Read the model definition and answer for the solid it produces. Units are mm, in the model's axes. Coordinates: 2 decimals unless noted, no trailing zeros. Order: outer loops, then holes, each group sorted by start corner. A loop starts at its lowest first (then second) coordinate and runs counter-clockwise, first axis right, second up. Notation, with made-up numbers: M 42,-6 L 79,-6 A34 ccw 79,31 Z; hole C 33.25,-26.75 d9. An arc over 180 degrees is marked long. One line per question, with ' | ' between items. Start each with the question number.
1) Consider probe 1 along Y at (x, z) = (0, 1.65); probe 2 along X at (y, z) = (-2.5, 1.5); probe 3 along X at (y, z) = (-3, 2.3). Determine where each line is inside the solid, lowest interval first.
2) Find section B-B, the plane x = 27. Write down the section's boundary in (y, z).
3) Find section A-A, the plane y = 33.5. Write down the section's boundary in (x, z), plus the area to 3 significant figures.
4) Find section C-C, the plane z = 1.45. Write down the section's boundary in (x, y).
5) Find section D-D, the plane y = -14.5. Write down the section's boundary in (x, z), plus the area to 3 significant figures.
6) Given P1, Ø16, axis at x = 27, y = 0, coming from the -Z side; P2, Ø1.5, axis at x = -8.5, z = 2, coming from the +Y side; P3, Ø1.5, axis at x = -7, z = 2, coming from the +Y side; P4, Ø1.5, axis at y = 10, z = 0.5, coming from the +X side, each flat-ended and moving along its own axis, determine where each tip first touches the part or whether it passes through.
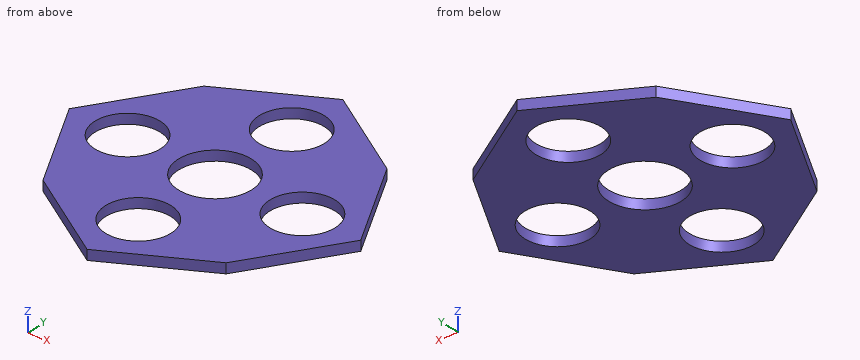
from build123d import *

# Parameters (mm, degrees)
F0_R     = 9.85
F0_R_2   = 11
F1_DEPTH = 3


with BuildPart() as f1:
    # F0 (on Top) → F1 (new body)
    with BuildSketch(Plane.XY):
        Polygon((-28.284271, 28.284271), (-45, 0), (-28.284271, -28.284271), (0, -45), (28.284271, -28.284271), (45, 0), (28.284271, 28.284271), (0, 45), align=None)
        with Locations((0, -27)):
            Circle(F0_R, mode=Mode.SUBTRACT)
        with Locations((-27, 0)):
            Circle(F0_R, mode=Mode.SUBTRACT)
        Circle(F0_R_2, mode=Mode.SUBTRACT)
        with Locations((27, 0)):
            Circle(F0_R, mode=Mode.SUBTRACT)
        with Locations((0, 27)):
            Circle(F0_R, mode=Mode.SUBTRACT)
    extrude(amount=F1_DEPTH)


solid = f1.part
Report:
1) probe 1: y = -45 to -36.85, -17.15 to -11, 11 to 17.15, 36.85 to 45 | probe 2: x = -43.52 to -36.53, -17.47 to -10.71, 10.71 to 17.47, 36.53 to 43.52 | probe 3: x = -43.23 to -36.38, -17.62 to -10.58, 10.58 to 17.62, 36.38 to 43.23
2) outline: M -29.04,0 L -9.85,0 L -9.85,3 L -29.04,3 Z; M 9.85,0 L 29.04,0 L 29.04,3 L 9.85,3 Z
3) outline: M -19.46,0 L -7.4,0 L -7.4,3 L -19.46,3 Z; M 7.4,0 L 19.46,0 L 19.46,3 L 7.4,3 Z | area: 72.3 mm^2
4) outline: M -45,0 L -28.28,-28.28 L 0,-45 L 28.28,-28.28 L 45,0 L 28.28,28.28 L 0,45 L -28.28,28.28 Z; hole C -27,0 d19.7; hole C 0,0 d22; hole C 0,-27 d19.7; hole C 0,27 d19.7; hole C 27,0 d19.7
5) outline: M -36.43,0 L 36.43,0 L 36.43,3 L -36.43,3 Z | area: 219 mm^2
6) P1: passes through | P2: stops at y = 40.42 | P3: stops at y = 41.31 | P4: stops at x = 39.53
